The listing builds one solid part. Answer for the finished solid, in the listing's coordinates (mm). A direction names the side the tool comes from. Coordinates: 2 decimals unless noted, no trailing zeros. Write each loop counter-clockwise with the first axis right and the second up, starting at its lowest first coordinate (ties: lowest second). Pieces come first, ordered by that corner, then holes. Notation, with made-up numbers: M 79.5,44 L 103.5,44 A11 cw 103.5,61 Z; hole C 29.25,11.25 d9. An arc over 180 degrees is marked long. Write item = value, one per line. Start each with the question number.
```python
from build123d import *

# Parameters (mm, degrees)
DODANIE_WYCI_GNI_CIE1_DEPTH = 10
SKORUPA1_T                  = -2
ZAOKR_GLENIE1_R             = 0.5
SZKIC2_R                    = 3
WYTNIJ_WYCI_GNI_CIE1_DEPTH  = 10


with BuildPart() as part:
    # Szkic1 → Dodanie-wyciągnięcie1 (new body, symmetric)
    with BuildSketch(Plane(origin=(0, 0, 0), x_dir=(0, 0, -1), z_dir=(1, 0, 0))):
        with BuildLine():
            Line((0, -25), (-20.857864376, -25))
            ThreePointArc((-20.857864376, -25), (-24.6846987, -24.238795325), (-27.928932188, -22.071067812))
            Line((-27.928932188, -22.071067812), (-37.071067812, -12.928932188))
            ThreePointArc((-37.071067812, -12.928932188), (-39.238795325, -9.6846987), (-40, -5.857864376))
            Line((-40, -5.857864376), (-40, 0))
            Line((-40, 0), (0, 0))
            ThreePointArc((0, 0), (-12.5, -12.5), (0, -25))
        make_face()
    extrude(amount=DODANIE_WYCI_GNI_CIE1_DEPTH, both=True)

    # Skorupa1
    skorupa1_openings = [part.faces().sort_by_distance(p)[0] for p in [
        (0, -25, 10.428932188),
        (0, -23.887164616, 24.539048491),
        (0, -17.5, 32.5),
        (0, -9.539048491, 38.887164616),
        (0, -2.928932188, 40),
        (0, -12.5, 6.25),
    ]]
    offset(amount=SKORUPA1_T, openings=skorupa1_openings, kind=Kind.INTERSECTION)

    # Zaokrąglenie1
    zaokr_glenie1_edges = [part.edges().sort_by_distance(p)[0] for p in [
        (-8, -2, 23.391164992),
        (8, -2, 23.391164992),
    ]]
    fillet(zaokr_glenie1_edges, radius=ZAOKR_GLENIE1_R)

    # Szkic2 → Wytnij-wyciągnięcie1 (cut)
    with BuildSketch(Plane(origin=(0, 0, 0), x_dir=(1, 0, 0), z_dir=(0, 1, 0))):
        with Locations((0, -27.5)):
            Circle(SZKIC2_R)
    extrude(amount=-WYTNIJ_WYCI_GNI_CIE1_DEPTH, mode=Mode.SUBTRACT)


solid = part.part
```
1. Each of these flat-tipped pins is pushed along its axis until it touches: pin 1 (10 mm diameter, centred on y = -8.5, z = 8, fed in from +X); pin 2 (1.5 mm diameter, centred on x = 7, y = -4.5, fed in from +Z); pin 3 (6 mm diameter, centred on x = -7.5, y = -12.5, fed in from -Z). Where does it stop, or does it pass through?
2. The part is cut by section B-B, the plane z = 27.5. Write down the section's boundary in (x, y).
3. For faces 1 (the face through (8, -14, 24)), 2 (the face through (9.014, -9.735, 39.218)), determine the directions among +Z, -Z, +X, -X, +Y, -Y from which every point of the face is accessible in a straight line to the end or side of a thin tool.
4. The part is cut by section D-D, the plane x = 8.5. Write down the section's boundary in (y, z), and give its area (3 significant figures).
5. Straight lines are drawn through the part: L1, parallel to X at y = -0.45, z = 27.5; L2, parallel to X at y = -23.25, z = 10; L3, parallel to Y at x = 6, z = 24. For each, find the intervals that lie inside material, in ascending order. Write a range as [from, to].
6. The part is cut by section C-C, the plane x = 2.5. Write down the section's boundary in (y, z).
7. The part is cut by section A-A, the plane y = -16.75. Write down the section's boundary in (x, z).
8. For a pull along Z with two mould halves and no side action, classify faces 3 (the face through (-9, -18, 32)), 4 (the face through (-0.65, -0.99, 30.43)), 5 (the face through (-8, -14, 24)), 6 (the face through (0.14, -1.54, 6.01)) as pulls with the +Z half, pulls with the -Z half, needs draft (parallel to the pull), parting line crosses it, or undercut.
Solution:
q1.pin_1 = 10
q1.pin_2 = through
q1.pin_3 = 12.14
q2.outline = M -10,-22.48 L -8,-22.48 L -8,-2.5 A0.5 cw -7.5,-2 L -3,-2 L -3,0 L -10,0 Z; M 3,-2 L 7.5,-2 A0.5 cw 8,-2.5 L 8,-22.48 L 10,-22.48 L 10,0 L 3,0 Z
q3.face_1 = +Z, -Z, -Y
q3.face_2 = +Z, +X, -X, -Y
q4.outline = M -25,0 A12.5 cw 0,0 L 0,40 L -5.86,40 A10 ccw -12.93,37.07 L -22.07,27.93 A10 ccw -25,20.86 Z
q4.area = 638 mm^2
q5.L1 = [-10, -3], [3, 10]
q5.L2 = [-10, -8], [8, 10]
q5.L3 = [-2, 0]
q6.outline = M -2,6.78 A12.5 cw 0,0 L 0,25.84 L -2,25.84 Z; M -2,29.16 L 0,29.16 L 0,40 L -2,40 Z
q7.outline = M -10,11.76 L -8,11.76 L -8,33.25 L -10,33.25 Z; M 8,11.76 L 10,11.76 L 10,33.25 L 8,33.25 Z
q8.face_3 = pulls with the +Z half
q8.face_4 = undercut
q8.face_5 = needs draft
q8.face_6 = pulls with the -Z half
